Build history of the part. All positions in model axes, mm. Face numbers are marked on the shaded views. A direction names the side the tool comes from. Coordinates: 2 decimals unless noted, no trailing zeros. Order: outer loops, then holes, each group sorted by start corner. A loop starts at its lowest first (then second) coordinate and runs counter-clockwise, first axis right, second up. Notation, with made-up numbers: (81.25, 44.25) - (115.25, 44.25) arc R11 cw to (115.25, 63.25) - close; hole circle Ø6 at (62, 10.5). An arc over 180 degrees is marked (long way). One line per item, written item: value.
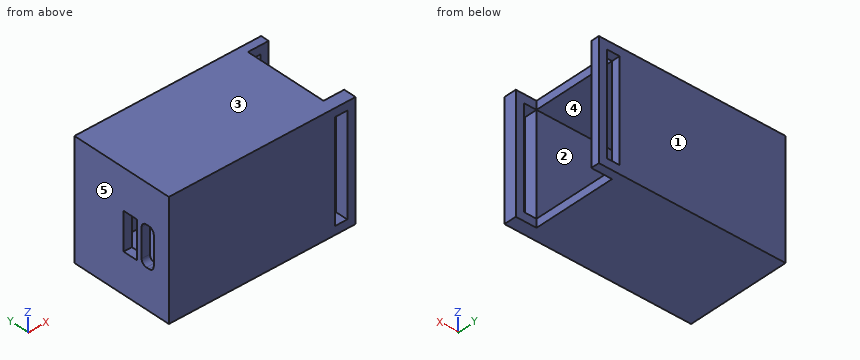
from build123d import *

# Parameters (mm, degrees)
SKETCH1_W           = 45
SKETCH1_H           = 28
BOSS_EXTRUDE1_DEPTH = 3
BOSS_EXTRUDE2_DEPTH = 22
SKETCH4_W           = 45
SKETCH4_H           = 28
SKETCH4_W_2         = 3
SKETCH4_H_2         = 24
BOSS_EXTRUDE4_DEPTH = 2
SKETCH5_W           = 9
SKETCH5_H           = 3.5
CUT_EXTRUDE1_DEPTH  = 2
SKETCH6_W           = 3
SKETCH6_H           = 24
CUT_EXTRUDE2_DEPTH  = 3


with BuildPart() as part:
    # Sketch1 → Boss-Extrude1 (new body)
    with BuildSketch(Plane(origin=(0, 0, 0), x_dir=(1, 0, 0), z_dir=(0, 1, 0))):
        with Locations((22.5, 14)):
            Rectangle(SKETCH1_W, SKETCH1_H)
    extrude(amount=BOSS_EXTRUDE1_DEPTH)

    # Sketch2 → Boss-Extrude2 (add)
    with BuildSketch(Plane(origin=(0, 3, 0), x_dir=(1, 0, 0), z_dir=(0, 1, 0))):
        Polygon((40, 26), (40, 28), (0, 28), (0, 0), (40, 0), (40, 2), (2, 2), (2, 26), align=None)
    extrude(amount=BOSS_EXTRUDE2_DEPTH)

    # Sketch4 → Boss-Extrude4 (add)
    with BuildSketch(Plane(origin=(0, 25, 0), x_dir=(1, 0, 0), z_dir=(0, 1, 0))):
        with Locations((22.5, 14)):
            Rectangle(SKETCH4_W, SKETCH4_H)
        with Locations((41.5, 14)):
            Rectangle(SKETCH4_W_2, SKETCH4_H_2, mode=Mode.SUBTRACT)
    extrude(amount=-BOSS_EXTRUDE4_DEPTH)

    # Sketch5 → Cut-Extrude1 (cut)
    with BuildSketch(Plane.ZY):
        with BuildLine():
            Line((-18.72, 5.25), (-18.72, 5.96))
            ThreePointArc((-18.72, 5.96), (-18.353883476, 6.843883476), (-17.47, 7.21))
            Line((-17.47, 7.21), (-10.53, 7.21))
            ThreePointArc((-10.53, 7.21), (-9.646116524, 6.843883476), (-9.28, 5.96))
            Line((-9.28, 5.96), (-9.28, 5.25))
            ThreePointArc((-9.28, 5.25), (-9.646116524, 4.366116524), (-10.53, 4))
            Line((-10.53, 4), (-17.47, 4))
            ThreePointArc((-17.47, 4), (-18.353883476, 4.366116524), (-18.72, 5.25))
        make_face()
        with Locations((-14, 10.25)):
            Rectangle(SKETCH5_W, SKETCH5_H)
    extrude(amount=-CUT_EXTRUDE1_DEPTH, mode=Mode.SUBTRACT)

    # Sketch6 → Cut-Extrude2 (cut)
    with BuildSketch(Plane(origin=(0, 3, 0), x_dir=(1, 0, 0), z_dir=(0, 1, 0))):
        with Locations((41.5, 14)):
            Rectangle(SKETCH6_W, SKETCH6_H)
    extrude(amount=-CUT_EXTRUDE2_DEPTH, mode=Mode.SUBTRACT)


solid = part.part
1. Band-saw the part on C-C, the plane z = -21.25. Give the cut face in (x, y).
Values found:
outline: (0, 0) - (40, 0) - (40, 3) - (2, 3) - (2, 23) - (40, 23) - (40, 25) - (0, 25) - close; (43, 0) - (45, 0) - (45, 3) - (43, 3) - close; (43, 23) - (45, 23) - (45, 25) - (43, 25) - close
2. Band-saw the part on D-D, the plane y = 23.75. Give the cut face in (x, z).
Values found:
outline: (0, -28) - (45, -28) - (45, 0) - (0, 0) - close; hole (40, -26) - (43, -26) - (43, -2) - (40, -2) - close
3. Two-plate mould, pull along Z, no slides. Class the marked faces 3, 4 and 5: pulls with the +Z half, pulls with the -Z half, needs draft (parallel to the pull), parting line crosses it, or undercut.
Values found:
face 3: pulls with the +Z half
face 4: undercut
face 5: needs draft
4. Probe line 1 along Y through (x, z) = (25.5, -12.75); line 2 along X through (y, z) = (2.25, -7.75); line 3 along Z through (x, y) = (13, 7). List the from-to ranges inside material, lowest first.
Values found:
line 1: y = 0 to 3, 23 to 25
line 2: x = 0 to 40, 43 to 45
line 3: z = -28 to -26, -2 to 0
5. Band-saw the part on A-A, the plane x = 17.5. Give the cut face in (y, z), and give its area (3 significant figures).
Values found:
outline: (0, -28) - (25, -28) - (25, 0) - (0, 0) - close; hole (3, -26) - (23, -26) - (23, -2) - (3, -2) - close
area: 220 mm2
6. Band-saw the part on B-B, the plane y = 11.5. Give the cut face in (x, z), and give its area (3 significant figures).
Values found:
outline: (0, -28) - (40, -28) - (40, -26) - (2, -26) - (2, -18.5) - (0, -18.5) - close; (0, -9.5) - (2, -9.5) - (2, -2) - (40, -2) - (40, 0) - (0, 0) - close
area: 190 mm2
7. Flat gauge pins, fed straight in: P1, Ø4, axis at y = 16.5, z = -22, coming from the +X side; P2, Ø1.6, axis at y = 8.5, z = -26.5, coming from the +X side. Where does each tip first touch, or does it go through?
Values found:
P1: stops at x = 2
P2: stops at x = 40
8. 3-axis set-ups, long thin cutter, end or side, ignore diameter. For the marked faces 1 and 2: which of +Z, -Z, +X, -X, +Y, -Y reach the whole face in a straight line?
Values found:
face 1: +Z, -Z, +X, -X, +Y
face 2: +X
